```python
from build123d import *

# Parameters (mm, degrees)
SKETCH1_R                                        = 3
BOSS_EXTRUDE1_DLUGOSC_CALKOWITA_S4_DEPTH         = 5
BOSS_EXTRUDE2_PRZEDLUZENIE_DO_MONTAZU_DEPTH      = 8
BOSS_EXTRUDE2_PRZEDLUZENIE_DO_MONTAZU_DEPTH_BACK = 13
SKETCH2_R                                        = 1.5


with BuildPart() as part:
    # Sketch1 → Boss-Extrude1 dlugosc calkowita S4 (new body)
    with BuildSketch(Plane.XY):
        Circle(SKETCH1_R)
    extrude(amount=BOSS_EXTRUDE1_DLUGOSC_CALKOWITA_S4_DEPTH)

    # Sketch2 → Boss-Extrude2 przedluzenie do montazu (add, two sides: drawn at the far end of the back side and taken through both)
    with BuildSketch(Plane(origin=(0, 0, 0), x_dir=(-1, 0, 0), z_dir=(0, 0, -1)).offset(-BOSS_EXTRUDE2_PRZEDLUZENIE_DO_MONTAZU_DEPTH_BACK)):
        Circle(SKETCH2_R)
    extrude(amount=BOSS_EXTRUDE2_PRZEDLUZENIE_DO_MONTAZU_DEPTH + BOSS_EXTRUDE2_PRZEDLUZENIE_DO_MONTAZU_DEPTH_BACK)


solid = part.part
```
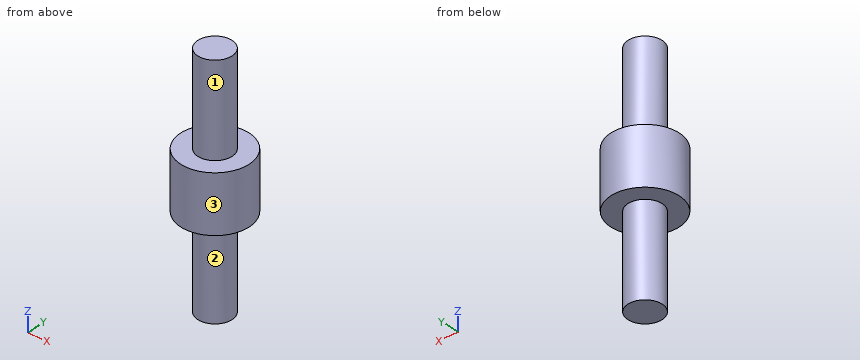
Input: part model. Units: mm. Frame: model coordinates. Face numbers are marked on the shaded views. A direction names the side the tool comes from. Coordinates: 2 decimals unless noted, no trailing zeros. Loops run counter-clockwise (first coordinate to the right, second up) from the corner with the lowest first, then second, coordinate; pieces in that order, holes last. Notation, with made-up numbers: M 50,-40 L 73,-40 A18 ccw 73,-15 Z; hole C -5,70 d4. An arc over 180 degrees is marked long. One line per item, written item: value.
(1) Reachability of the marked faces 1, 2 and 3 from +Z, -Z, +X, -X, +Y, -Y: full face, straight path, thin tool, end or side. Return the list, or none.
Filled in:
face 1: +Z
face 2: -Z
face 3: +Z, -Z
(2) Section C-C (z = -5.75). Output: boundary loops of the cut face in (x, y).
Filled in:
outline: C 0,0 d3
(3) Line query: line 1 along Z through (x, y) = (0.1, -2.8); line 2 along X through (y, z) = (0.1, 8); line 3 along Y through (x, z) = (-0.35, 9.75). Output: solid intervals per line, ascending. Write a range as from..to.
Filled in:
line 1: 0..5
line 2: -1.5..1.5
line 3: -1.46..1.46
(4) Section D-D (x = 1.8). Output: boundary loops of the cut face in (y, z), and give its area (3 significant figures).
Filled in:
outline: M -2.4,0 L 2.4,0 L 2.4,5 L -2.4,5 Z
area: 24.0 mm^2
(5) Section A-A (y = 0). Output: boundary loops of the cut face in (x, z).
Filled in:
outline: M -3,0 L -1.5,0 L -1.5,-8 L 1.5,-8 L 1.5,0 L 3,0 L 3,5 L 1.5,5 L 1.5,13 L -1.5,13 L -1.5,5 L -3,5 Z
(6) Pin query (flat end, axial travel): pin 1 (3 mm diameter, centred on x = 2, z = 11, fed in from +Y). Return the tip coordinate at first contact, or that it passes through.
Filled in:
pin 1: y = 1.41
